Check sheet for the modelled part. Datum: model origin and axes. Units: mm. Face numbers are marked on the shaded views. A direction names the side the tool comes from. Round coordinates to 2 decimals unless told otherwise and drop trailing zeros. Order: outer loops, then holes, each group sorted by start corner. A loop starts at its lowest first (then second) coordinate and runs counter-clockwise, first axis right, second up.
Q1. Cross-section at A-A on x = -10.5. Record the cut outline in (y, z).
Q2. Mould release check, pull along Z, two halves, no side actions. Record for the marked faces 1, 2, 3 and 4: +Z half, -Z half, draft (parallel to the pull), parting line (faces both ways), or undercut.
Q3. Set-up check for the marked faces 5, 6, 7 and 8: record each of +Z, -Z, +X, -X, +Y, -Y from which the full face is reachable in a straight line by a thin tool's end or side.
Q4. Cross-section at C-C on y = -6. Record the cut outline in (x, z).
Q5. Depth check by flat-ended pin: P1, Ø1, axis at y = -9.5, z = -5, coming from the +X side; P2, Ø3, axis at x = -9.5, y = -7.5, coming from the -Z side; P3, Ø5.5, axis at x = 0, y = 0, coming from the -Z side; P4, Ø1.5, axis at x = 2, y = -6.5, coming from the -Z side. Enter the tip coordinate at first touch or a pass-through.
Q6. Cross-section at B-B on y = 12.45. Record the cut outline in (x, z), then the cut area to 3 significant figures.
Q7. Scan lines: probe 1 along Y at (x, z) = (10.5, 0.4); probe 2 along Y at (x, z) = (1.5, -0.75); probe 3 along Y at (x, z) = (-7.5, -2.5). Record each from-to range of solid material in increasing order.
Q8. Cross-section at D-D on z = -5.5. Record the cut outline in (x, y).
Autodesk Inventor part; units mm, degrees
ref_plane "YZ Plane" through (0, 0, 0) normal (1, 0, 0) x (0, 1, 0)
ref_plane "XZ Plane" through (0, 0, 0) normal (0, 1, 0) x (-1, 0, 0)
ref_plane "XY Plane" through (0, 0, 0) normal (0, 0, 1) x (1, 0, 0)
sketch "スケッチ1" plane through (0, 0, 0) normal (0, 0, 1) x (1, 0, 0)
  line L0 (-12.7, 14.45) -> (12.7, 14.45)
  line L1 (12.7, 14.45) -> (12.7, -9.55)
  line L2 (12.7, -9.55) -> (-12.7, -9.55)
  line L3 (-12.7, -9.55) -> (-12.7, 14.45)
  line L4 (-12.7, 14.45) -> (12.7, -9.55) construction
  line L5 (12.7, 14.45) -> (-12.7, -9.55) construction
  point P0 (0, 0)
  point P1 (0, 2.45)
  dimension "d0" = 25.4
  dimension "d1" = 24
  dimension "d2" = 14.45
extrude "押し出し1" add sketch "スケッチ1" along normal blind 1
sketch "スケッチ2" plane through (0, 0, 1) normal (0, 0, 1) x (1, 0, 0)
  line L0 (4.25, 4.25) -> (-4.25, 4.25)
  line L1 (-4.25, 4.25) -> (-4.25, -4.25)
  line L2 (-4.25, -4.25) -> (4.25, -4.25)
  line L3 (4.25, -4.25) -> (4.25, 4.25)
  line L4 (4.25, 4.25) -> (-4.25, -4.25) construction
  line L5 (-4.25, 4.25) -> (4.25, -4.25) construction
  point P0 (0, 0)
  dimension "d5" = 8.5
extrude "押し出し2" add sketch "スケッチ2" along normal blind 3.5
sketch "スケッチ3" plane through (0, 0, 4.5) normal (0, 0, 1) x (1, 0, 0)
  circle A0 centre (0, 0) radius 3.65
  dimension "d8" = 7.3
extrude "押し出し3" add sketch "スケッチ3" along normal blind 2.4
sketch "スケッチ4" plane through (0, 0, 6.9) normal (0, 0, 1) x (1, 0, 0)
  circle A0 centre (0, 0) radius 3
  dimension "d11" = 6
extrude "押し出し4" cut sketch "スケッチ4" against normal blind 0.5
sketch "スケッチ5" plane through (0, 0, 1) normal (0, 0, 1) x (1, 0, 0)
  line L0 (10.5, -0.05) -> (-10.5, -0.05) construction
  line L1 (-10.5, -0.05) -> (-10.5, 12.45) construction
  line L2 (-10.5, 12.45) -> (10.5, 12.45) construction
  line L3 (10.5, 12.45) -> (10.5, -0.05) construction
  line L4 (10.5, -0.05) -> (-10.5, 12.45) construction
  line L5 (-10.5, -0.05) -> (10.5, 12.45) construction
  line L6 (12.7, 14.45) -> (-12.7, 14.45)
  circle A0 centre (-10.5, 12.45) radius 1.1
  circle A1 centre (10.5, 12.45) radius 1.1
  circle A2 centre (-10.5, -0.05) radius 1.1
  circle A3 centre (10.5, -0.05) radius 1.1
  point P0 (0, 0)
  point P1 (0, 6.2)
  dimension "d14" = 21
  dimension "d15" = 12.5
  dimension "d16" = 2
  dimension "d17" = 2.2
extrude "押し出し5" cut sketch "スケッチ5" against normal through all
sketch "スケッチ6" plane through (0, 0, 0) normal (0, 0, -1) x (-1, 0, 0)
  line L0 (10, -4.55) -> (-10, -4.55)
  line L1 (-10, -4.55) -> (-10, -9.55)
  line L2 (-10, -9.55) -> (10, -9.55)
  line L3 (10, -9.55) -> (10, -4.55)
  line L4 (10, -4.55) -> (-10, -9.55) construction
  line L5 (-10, -4.55) -> (10, -9.55) construction
  line L6 (12.7, -9.55) -> (-12.7, -9.55)
  point P0 (0, 0)
  point P1 (0, -7.05)
  dimension "d20" = 20
  dimension "d21" = 5
extrude "押し出し6" add sketch "スケッチ6" along normal blind 3
sketch "スケッチ7" plane through (0, 0, 0) normal (0, 0, -1) x (-1, 0, 0)
  line L0 (8.5, 1.2) -> (-8.5, 1.2)
  line L1 (-8.5, 1.2) -> (-8.5, 11.2)
  line L2 (-8.5, 11.2) -> (8.5, 11.2)
  line L3 (8.5, 11.2) -> (8.5, 1.2)
  line L4 (8.5, 1.2) -> (-8.5, 11.2) construction
  line L5 (-8.5, 1.2) -> (8.5, 11.2) construction
  circle A0 centre (-10.5, 12.45) radius 1.1
  circle A1 centre (-10.5, -0.05) radius 1.1
  point P0 (0, 0)
  point P1 (0, 6.2)
  dimension "d24" = 17
  dimension "d25" = 10
  dimension "d26" = 6.25
  dimension "d27" = 6.25
extrude "押し出し7" add sketch "スケッチ7" along normal blind 1 contours L0 L1 L2 L3
sketch "スケッチ8" plane through (10, -9.55, 0) normal (1, 0, 0) x (0, 0, -1)
  line L0 (1.6, -2) -> (1.4, -2) construction
  line L1 (1.4, -2) -> (1.4, 0)
  line L2 (1.4, 0) -> (1.6, 0)
  line L3 (1.6, 0) -> (1.6, -2)
  line L4 (1.6, -2) -> (1.4, 0) construction
  line L5 (1.4, -2) -> (1.6, 0) construction
  line L6 (0, 0) -> (3, 0)
  circle A0 centre (5.5, -2) radius 4 construction
  line L7 (1.5, 0) -> (1.5, -2) construction
  circle A1 centre (5.5, -2) radius 4.1
  circle A2 centre (5.5, -2) radius 3.9
  arc A3 (1.4, 11) -> (7.2575, 1.4815) centre (12.0625, 11) ccw
  line L8 (1.4, 0) -> (1.4, 9.037) construction
  line L9 (1.6, 0) -> (1.6, 10.1272) construction
  arc A4 (1.6, 11) -> (7.3476, 1.6601) centre (12.0625, 11) ccw
  line L10 (1.4, 11) -> (1.6, 11)
  point P0 (0, 9.55)
  point P1 (1.5, -1)
  dimension "d30" = 0.2
  dimension "d31" = 2
  dimension "d32" = 8
  dimension "d33" = 11
extrude "押し出し8" add sketch "スケッチ8" against normal up to surface (20 mm away) contours A1 L3 A2 A3 | L1 L2 L3 A1 | A1 A3 L10 A4
sketch "スケッチ9" plane through (0, 0, 1) normal (0, 0, 1) x (1, 0, 0)
  line L0 (-3.5, 11.25) -> (3.5, 11.25)
  line L1 (3.5, 11.25) -> (3.5, 4.25)
  line L2 (3.5, 4.25) -> (-3.5, 4.25)
  line L3 (-3.5, 4.25) -> (-3.5, 11.25)
  line L4 (-3.5, 11.25) -> (3.5, 4.25) construction
  line L5 (3.5, 11.25) -> (-3.5, 4.25) construction
  line L6 (-4.25, 4.25) -> (4.25, 4.25)
  line L7 (3.5, 11.25) -> (-6.5, 11.25)
  line L8 (-6.5, 11.25) -> (-6.5, 7.25)
  line L9 (-6.5, 7.25) -> (3.5, 7.25)
  line L10 (3.5, 7.25) -> (3.5, 11.25)
  point P0 (0, 0)
  point P1 (0, 7.75)
  point P2 (-3.5, 7.25)
  dimension "d65" = 7
  dimension "d66" = 7
  dimension "d67" = 10
  dimension "d68" = 4
extrude "押し出し9" add sketch "スケッチ9" along normal blind 1.5
properties part number "cam"
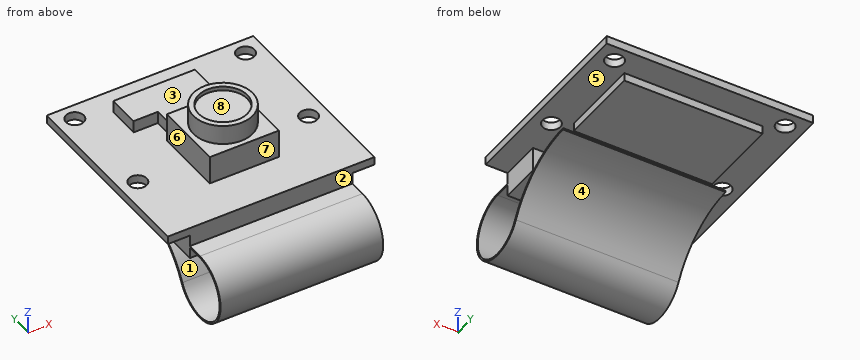
Results found:
1. outline: (-9.55, 0) - (-1.15, 0) - (-1.15, 1) - (-9.55, 1) - close; (1.05, 0) - (11.35, 0) - (11.35, 1) - (1.05, 1) - close; (13.55, 0) - (14.45, 0) - (14.45, 1) - (13.55, 1) - close
2. face 1: undercut
2. face 2: draft
2. face 3: +Z half
2. face 4: -Z half
3. face 5: none
3. face 6: +Z, -X, -Y
3. face 7: +Z, +X, -X, -Y
3. face 8: +Z
4. outline: (-12.7, 0) - (-10, 0) - (-10, -3) - (10, -3) - (10, 0) - (12.7, 0) - (12.7, 1) - (-12.7, 1) - close; (-10, -4.72) - (10, -4.72) - (10, -4.43) - (-10, -4.43) - close
5. P1: passes through
5. P2: stops at z = -8.71
5. P3: stops at z = -2.48
5. P4: stops at z = -6.25
6. outline: (-12.7, 0) - (-11.6, 0) - (-11.6, 1) - (-12.7, 1) - close; (-9.4, 0) - (9.4, 0) - (9.4, 1) - (-9.4, 1) - close; (11.6, 0) - (12.7, 0) - (12.7, 1) - (11.6, 1) - close
6. area: 21.0 mm2
7. probe 1: y = -9.55 to -1.15, 1.05 to 11.35, 13.55 to 14.45
7. probe 2: y = -9.55 to -4.55, 1.2 to 11.2
7. probe 3: y = -14.34 to -14.04, -9.55 to -4.55, -3.27 to -2.8
8. outline: (-10, -15.65) - (10, -15.65) - (10, -15.45) - (-10, -15.45) - close; (-10, -6.95) - (10, -6.95) - (10, -6.7) - (-10, -6.7) - close
